from build123d import *

# Parameters (mm, degrees)
F1_DEPTH        = 41.25
F0_W            = 6.25
F0_H            = 30
F2_DEPTH        = 25.25
F3_START        = 6
F2_FACE_W       = 6.25
F2_FACE_H       = 30
F3_DEPTH        = 10
F4_START        = 6.25
F4_DEPTH        = 25
F5_START        = 35
F5_DEPTH        = 6.25
F6_DEPTH        = 6.25
F7_W            = 175
F7_H            = 16.25
F8_DEPTH        = 10
F7_W_2          = 187.5
F7_H_2          = 28.75
F9_DEPTH        = 3
F11_D           = 3
F11_DEPTH       = 12
F11_CSINK_D     = 5
F11_CSINK_ANGLE = 90
F11_TIP         = 0.9012909285


with BuildPart() as f1:
    # F0 (on Top) → F1 (new body)
    with BuildSketch(Plane.XY):
        Polygon((0, -100), (0, 100), (-75, 100), (-75, 46), (-75, 33.5), (-75, 15), (-68.75, 15), (-68.75, 93.75), (-6.25, 93.75), (-6.25, -93.75), (-68.75, -93.75), (-68.75, -15), (-75, -15), (-75, -33.5), (-75, -46), (-75, -100), align=None)
    extrude(amount=F1_DEPTH)

    # F0 (on Top) → F2 (join)
    with BuildSketch(Plane.XY):
        with Locations((-71.875, 0)):
            Rectangle(F0_W, F0_H)
    extrude(amount=F2_DEPTH)

    # F2_face (on face) → F3 (join)
    with BuildSketch(Plane(origin=(-71.875, 0, 25.25), x_dir=(1, 0, 0), z_dir=(0, 0, 1)).offset(F3_START)):
        Rectangle(F2_FACE_W, F2_FACE_H)
    extrude(amount=F3_DEPTH)

    # F0 (on Top) → F4 (join)
    with BuildSketch(Plane.XY.offset(F4_START)):
        Polygon((-75, 33.5), (-75, 46), (-87.5, 46), (-87.5, 51), (-92.5, 51), (-92.5, 28.5), (-87.5, 28.5), (-87.5, 33.5), align=None)
        Polygon((-87.5, -46), (-75, -46), (-75, -33.5), (-87.5, -33.5), (-87.5, -28.5), (-92.5, -28.5), (-92.5, -51), (-87.5, -51), align=None)
    extrude(amount=F4_DEPTH)

    # F0 (on Top) → F5 (join)
    with BuildSketch(Plane.XY.offset(F5_START)):
        Polygon((-68.75, 93.75), (-68.75, 15), (-68.75, -15), (-68.75, -93.75), (-6.25, -93.75), (-6.25, 93.75), align=None)
    extrude(amount=F5_DEPTH)

    # F0 (on Top) → F6 (join)
    with BuildSketch(Plane.XY):
        Polygon((-68.75, 93.75), (-68.75, 15), (-68.75, -15), (-68.75, -93.75), (-6.25, -93.75), (-6.25, 93.75), align=None)
    extrude(amount=F6_DEPTH)

    # F7 (on face) → F8 (cut)
    with BuildSketch(Plane.YZ):
        with Locations((0, 20.625)):
            Rectangle(F7_W, F7_H)
    extrude(amount=-F8_DEPTH, mode=Mode.SUBTRACT)

    # F7 (on face) → F9 (cut)
    with BuildSketch(Plane.YZ):
        with Locations((0, 20.625)):
            Rectangle(F7_W_2, F7_H_2)
        with Locations((0, 20.625)):
            Rectangle(F7_W, F7_H, mode=Mode.SUBTRACT)
    extrude(amount=-F9_DEPTH, mode=Mode.SUBTRACT)

    # F11
    with Locations(Plane.YZ.offset(-3)):
        with Locations((-90.625, 31.875), (0, 31.875), (90.625, 31.875), (90.625, 9.375), (0, 9.375), (-90.625, 9.375)):
            CounterSinkHole(F11_D / 2, F11_CSINK_D / 2, depth=F11_DEPTH, counter_sink_angle=F11_CSINK_ANGLE)
            with Locations((0, 0, -(F11_DEPTH + F11_TIP / 2))):  # 118° drill point
                Cone(0, F11_D / 2, F11_TIP, mode=Mode.SUBTRACT)


solid = f1.part
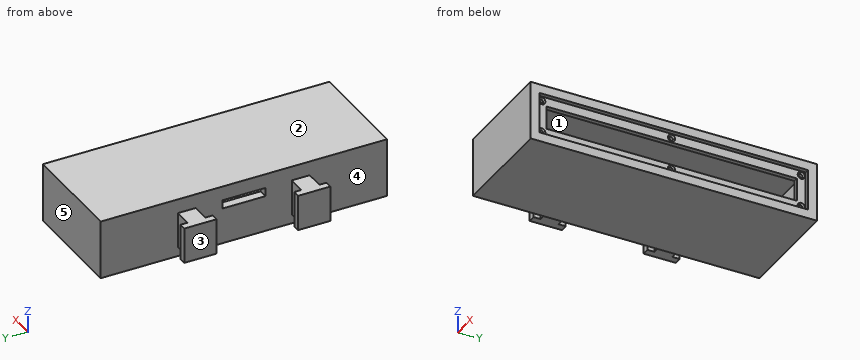
Check sheet for the modelled part. Datum: model origin and axes. Units: mm. Face numbers are marked on the shaded views. A direction names the side the tool comes from. Coordinates: 2 decimals unless noted, no trailing zeros. Loops run counter-clockwise (first coordinate to the right, second up) from the corner with the lowest first, then second, coordinate; pieces in that order, holes last. Notation, with made-up numbers: (70, 17.25) -> (79, 17.25) arc R36 ccw to (79, 52.25) -> close; hole circle Ø8 at (-18.75, -14). An arc over 180 degrees is marked (long way). Answer in a Markdown table with one row per item.
1. Sectioned sample at B-B, the plane x = -49. Record the boundary of the cut face in (y, z), then the cut area to 3 significant figures.
Check values:
| item | result |
|---|---|
| outline | (-100, 0) -> (100, 0) -> (100, 41.25) -> (-100, 41.25) -> close; hole (-93.75, 6.25) -> (93.75, 6.25) -> (93.75, 35) -> (-93.75, 35) -> close |
| area | 2,860 mm2 |
2. Access from +Z, -Z, +X, -X, +Y, -Y to the whole of each face (thin tool, end or side, straight path). Record for the marked faces 1 and 2.
Check values:
| item | result |
|---|---|
| face 1 | none |
| face 2 | +Z, +X, -X, +Y, -Y |
3. Go/stop test with flat-tipped pins: pin 1 (23 mm diameter, centred on y = 9, z = 15.5, fed in from +X); pin 2 (9 mm diameter, centred on x = -81.5, y = 36.5, fed in from -Z); pin 3 (2 mm diameter, centred on y = 45, z = 20, fed in from +X); pin 4 (12 mm diameter, centred on y = -20.5, z = 32, fed in from -X). Record where each tip stops, or that it passes through.
Check values:
| item | result |
|---|---|
| pin 1 | stops at x = 0 |
| pin 2 | stops at z = 6.25 |
| pin 3 | stops at x = -68.75 |
| pin 4 | stops at x = -75 |
4. Sectioned sample at A-A, the plane y = 64.5. Record the boundary of the cut face in (x, z).
Check values:
| item | result |
|---|---|
| outline | (-75, 0) -> (0, 0) -> (0, 6.25) -> (-3, 6.25) -> (-3, 12.5) -> (-6.25, 12.5) -> (-6.25, 6.25) -> (-68.75, 6.25) -> (-68.75, 35) -> (-6.25, 35) -> (-6.25, 28.75) -> (-3, 28.75) -> (-3, 35) -> (0, 35) -> (0, 41.25) -> (-75, 41.25) -> close |
5. Release check for a two-part mould opening along Y. For the marked faces 3, 4 and 5 record: released by +Y, released by -Y, zero draft, split by the parting line, or undercut.
Check values:
| item | result |
|---|---|
| face 3 | zero draft |
| face 4 | undercut |
| face 5 | released by +Y |
6. Material ranges on line 1 along X through (y, z) = (-81, 6.5); line 2 along Z through (x, y) = (-5, 0) (3 decimals); line 3 along Y through (x, z) = (-68, 33), recorded low to high. Write a range as [from, to].
Check values:
| item | result |
|---|---|
| line 1 | x = [-75, -68.75], [-6.25, -3] |
| line 2 | z = [0, 7.875], [10.875, 12.5], [28.75, 30.375], [33.375, 41.25] |
| line 3 | y = [-100, -93.75], [93.75, 100] |
